```python
from build123d import *

# Parameters (mm, degrees)
ESTRUSIONE_ESTRUSIONE1_DEPTH = 18


with BuildPart() as part:
    # Schizzo1 → Estrusione-Estrusione1 (new body)
    with BuildSketch(Plane.XY):
        with BuildLine():
            Line((0.437175512, -19.879120879), (11.437175512, -19.879120879))
            Line((11.437175512, -19.879120879), (11.437175512, 16.120879121))
            Line((11.437175512, 16.120879121), (-28.562824488, 16.120879121))
            Line((-28.562824488, 16.120879121), (-28.562824488, -19.879120879))
            Line((-28.562824488, -19.879120879), (-17.562824488, -19.879120879))
            Line((-17.562824488, -19.879120879), (-17.562824488, -1.681318681))
            ThreePointArc((-17.562824488, -1.681318681), (-14.387824488, 1.493681319), (-11.212824488, -1.681318681))
            Line((-11.212824488, -1.681318681), (-5.912824488, -1.681318681))
            ThreePointArc((-5.912824488, -1.681318681), (-2.737824488, 1.493681319), (0.437175512, -1.681318681))
            Line((0.437175512, -1.681318681), (0.437175512, -19.879120879))
        make_face()
    extrude(amount=ESTRUSIONE_ESTRUSIONE1_DEPTH)


solid = part.part
```
Here's how the part is built. I have some questions about the finished solid (model axes, mm). A direction names the side the tool comes from. Coordinates: 2 decimals unless noted, no trailing zeros. Order: outer loops, then holes, each group sorted by start corner. A loop starts at its lowest first (then second) coordinate and runs counter-clockwise, first axis right, second up. Notation, with made-up numbers: (-9, 72) - (24, 72) arc R20 cw to (24, 88) - close; hole circle Ø1 at (40.25, 6.25). An arc over 180 degrees is marked (long way). One line per question, with ' | ' between items.
(1) Suppose I cut it at C-C on x = -17. List the corners of the cut face in (y, z) for me.
Report:
outline: (0.12, 0) - (16.12, 0) - (16.12, 18) - (0.12, 18) - close
(2) Suppose I cut it at D-D on x = -1. List the corners of the cut face in (y, z) for me, and give its area (3 significant figures).
Report:
outline: (0.98, 0) - (16.12, 0) - (16.12, 18) - (0.98, 18) - close | area: 273 mm2
(3) Suppose I cut it at B-B on z = 8.5. List the corners of the cut face in (x, y) for me (3 decimals).
Report:
outline: (-28.563, -19.879) - (-17.563, -19.879) - (-17.563, -1.681) arc R3.175 cw to (-11.213, -1.681) - (-5.913, -1.681) arc R3.175 cw to (0.437, -1.681) - (0.437, -19.879) - (11.437, -19.879) - (11.437, 16.121) - (-28.563, 16.121) - close
(4) Will this pin go through, and if not, where does the flat tip stop? pin 1 (5 mm diameter, centred on x = -12, z = 11.5, fed in from -Y).
Report:
pin 1: stops at y = -1.68
(5) If I drill on L1, parallel to X at y = -1.5, z = 12; L2, parallel to X at y = -7, z = 4; L3, parallel to Y at x = -8, z = 14.25, over which ranges is the centre line in solid material (lowest first)?
Report:
L1: x = -28.56 to -17.56, -11.22 to -5.91, 0.43 to 11.44 | L2: x = -28.56 to -17.56, 0.44 to 11.44 | L3: y = -1.68 to 16.12
(6) If we mould it in two halves opening along X, with no side actions, what happens to faces 3 (the flat face through (-17.563, -11, 9)), 4 (the flat face through (11.437, -2, 9)), 5 (the flat face through (-9, 2, 18))? For each: pulls with the +X half, pulls with the -X half, needs draft (parallel to the pull), parting line crosses it, or undercut.
Report:
face 3: undercut | face 4: pulls with the +X half | face 5: needs draft
(7) For faces 1 (the flat face through (0.437, -11, 9)), 2 (the flat face through (-28.563, -2, 9)), which set-ups out of +Z, -Z, +X, -X, +Y, -Y let a thin tool reach every point of the face, with its end or its side?
Report:
face 1: +Z, -Z, -Y | face 2: +Z, -Z, -X, +Y, -Y
(8) Suppose I cut it at A-A on y = -17. List the corners of the cut face in (x, z) for me, and give its area (3 significant figures).
Report:
outline: (-28.56, 0) - (-17.56, 0) - (-17.56, 18) - (-28.56, 18) - close; (0.44, 0) - (11.44, 0) - (11.44, 18) - (0.44, 18) - close | area: 396 mm2
